Part model, mm, in its own coordinate system. A direction names the side the tool comes from. Give positions to 0.01 mm unless a question says otherwise; leave off trailing zeros. Write each loop counter-clockwise with the first axis right and the second up, starting at its lowest first coordinate (ties: lowest second). Pieces come first, ordered by that corner, then holes.
```python
from build123d import *

# Parameters (mm, degrees)
EXTRUDE_1_DEPTH = 0.3
SKETCH_3_W      = 1.8
SKETCH_3_H      = 0.3
EXTRUDE_2_DEPTH = 2
FILLET_1_R      = 0.3


with BuildPart() as part:
    # 草图1 → 凸台-拉伸1 (new body)
    with BuildSketch(Plane(origin=(0, 0, 0), x_dir=(0, 0, -1), z_dir=(1, 0, 0))):
        Polygon((-5.5, -2), (-5.5, -1.5), (-5.5, -0.5), (-5.5, 0.5), (-5.5, 1.5), (-5.5, 2), (5.5, 2), (5.5, 1.5), (5.5, 0.5), (5.5, -0.5), (5.5, -1.5), (5.5, -2), (-3.7, -2), (-3.7, -8.98), (-5.5, -8.98), align=None)
    extrude(amount=EXTRUDE_1_DEPTH)

    # 草图3 → 凸台-拉伸2 (add)
    with BuildSketch(Plane.ZY):
        with Locations((4.6, -8.83)):
            Rectangle(SKETCH_3_W, SKETCH_3_H)
    extrude(amount=EXTRUDE_2_DEPTH)

    # 圆角1
    fillet_1_edges = [part.edges().sort_by_distance(p)[0] for p in [
        (0.15, -2, -5.5),
        (0.15, 2, 5.5),
        (0.15, 2, -5.5),
    ]]
    fillet(fillet_1_edges, radius=FILLET_1_R)


solid = part.part
```
1) Wall check: L1, parallel to Y at x = -0.45, z = 4.75; L2, parallel to X at y = -1, z = 1.5; L3, parallel to Z at x = 0.25, y = -4.25. Give the ranges that are in metal, low to high.
Answers follow:
L1: y = -8.98 to -8.68
L2: x = 0 to 0.3
L3: z = 3.7 to 5.5
2) Pin check, flat tips, straight feed: pin 1 Ø3 at (y, z) = (-4.5, 1) entering from -X (3 decimals); pin 2 Ø3 at (y, z) = (-2, -1.5) entering from -X; pin 3 Ø0.5 at (x, z) = (-0.5, 5) entering from +Y. Stop position of each tip, or through.
Answers follow:
pin 1: passes through
pin 2: stops at x = 0
pin 3: stops at y = -8.68
3) 3-axis set-ups, long thin cutter, end or side, ignore diameter. For faces 1 (the face through (-1, -8.98, 5)), 2 (the face through (0, -1, 1)): which of +Z, -Z, +X, -X, +Y, -Y reach the whole face in a straight line?
Answers follow:
face 1: +Z, -Z, +X, -X, -Y
face 2: +Z, -Z, -X, +Y
4) Saw through at C-C, the plane x = -0.5. Write the cut outline in (y, z).
Answers follow:
outline: (-8.98, 3.7) - (-8.68, 3.7) - (-8.68, 5.5) - (-8.98, 5.5) - close
5) Saw through at A-A, the plane z = 4.75. Write the cut outline in (x, y).
Answers follow:
outline: (-2, -8.98) - (0.3, -8.98) - (0.3, 2) - (0, 2) - (0, -8.68) - (-2, -8.68) - close
6) Saw through at B-B, the plane y = -3.25. Write the cut outline in (x, z), then the cut area to 3 significant figures.
Answers follow:
outline: (0, 3.7) - (0.3, 3.7) - (0.3, 5.5) - (0, 5.5) - close
area: 0.540 mm2
